Here's how the part is built. I have some questions about the finished solid (model axes, mm). A direction names the side the tool comes from. Round coordinates to 2 decimals unless told otherwise and drop trailing zeros. Write each loop counter-clockwise with the first axis right and the second up, starting at its lowest first coordinate (ties: lowest second). Pieces come first, ordered by that corner, then holes. Notation, with made-up numbers: (21, 15) -> (76, 15) arc R33 ccw to (76, 45) -> close; hole circle Ø3 at (3.25, 70.25). An arc over 180 degrees is marked (long way). Put each result on its own line as item: value. Start each with the question number.
1. Suppose I cut it at A-A (y = 0). Please give me the cut outline in (x, z), then the cut area to 3 significant figures.
2. I need wall thicknesses on probe 1 along X at (y, z) = (0, 2.5); probe 2 along X at (y, z) = (-3.5, -7.5); probe 3 along Z at (x, y) = (7.5, -0.25). Which ranges of each line are inside material? Lowest first, please. Write a range as from..to.
3. Suppose I cut it at D-D (x = 11.5). Please give me the cut outline in (y, z).
4. Suppose I cut it at B-B (z = 0). Please give me the cut outline in (x, y), then the cut area to 3 significant figures.
5. Suppose I cut it at C-C (x = 29). Please give me the cut outline in (y, z), then the cut area to 3 significant figures.
6. For pin 1 (5 mm diameter, centred on x = 8.5, y = -5, fed in from +Z); pin 2 (3 mm diameter, centred on x = 17, z = -2.5, fed in from +Y); pin 3 (5 mm diameter, centred on y = 10, z = -9.5, fed in from +X); pin 4 (2.5 mm diameter, centred on x = 29, y = 0, fed in from +Z), each with a flat end and sliding along its axis, tell me the tip position at first contact or that it passes through.
7. Which directions (+Z, -Z, +X, -X, +Y, -Y) give clear straight access to the entire face, cutting with the end or side of a thin tool? Please do faces 1 (the face through (-4.5, 0, 0)), 2 (the face through (16.22, 3.69, -7.1)).
Autodesk Inventor part; units mm, degrees
ref_plane "Work Plane1" through (17.5, 0, 8) normal (0, 0, 1) x (1, 0, 0)
ref_plane "YZ Plane" through (0, 0, 0) normal (1, 0, 0) x (0, 1, 0)
ref_plane "XZ Plane" through (0, 0, 0) normal (0, 1, 0) x (-1, 0, 0)
sketch "Sketch1" plane through (0, 0, 0) normal (0, 0, 1) x (1, 0, 0)
  line L0 (-4.5, 0) -> (-4.5, 12.5)
  line L1 (-4.5, 12.5) -> (0, 12.5)
  line L2 (0, 12.5) -> (0, 8)
  line L3 (0, 8) -> (35, 8)
  line L4 (35, 8) -> (35, 0)
  line L5 (-4.5, 0) -> (35, 0)
  line L6 (-4, 0) -> (17, 0)
  line L7 (0, -0.98) -> (0, 3.08)
  circle A0 centre (29, 0) radius 2
  dimension "d0" = 16
  dimension "d1" = 25
  dimension "d2" = 4.5
  dimension "d3" = 35
  dimension "d5" = 6
  dimension "d6" = 4
revolve "Body" add sketch "Sketch1" angle 360 about axis through (-4.5, 0, 0) along (1, 0, 0) picked at (28.3903, 0.4694) contours L0 L1 L2 L3 L4 L5 A0 | A0 L5
extrude "Hole" cut sketch "Sketch1" along normal through all both and the other way through all contours A0 L5 | L5 A0
chamfer "Chamfer1" distance 1.6 angle 45 1 edges at (-4.5, -12.5, 0) measured on face at (-3, 12.4595, -1.0058)
chamfer "Chamfer2" distance 3 angle 30 1 edges at (35, -8, 0) measured on face at (11.6667, 7.9741, -0.6437)
ref_plane "Work Plane1" through (17.5, 0, 8) normal (0, 0, 1) x (1, 0, 0)
equation "\"d0\" = NND"
equation "\"d1\" = KOD"
equation "\"d2\" = KOH"
equation "\"d3\" = NLG"
equation "\"d5\" = DIST"
equation "\"d6\" = BOR"
equation "\"d7\" = NND"
equation "\"d9\" = PHH2"
equation "\"d10\" = FAWI2"
equation "\"d16\" = PHH2"
equation "\"d11\" = PHH1"
equation "\"d12\" = FAWI1"
equation "\"d17\" = PHH1"
equation "\"PHH1\" = 3"
equation "\"PHH2\" = 1.6"
equation "\"KOD\" = 25"
equation "\"KOH\" = 4.5"
equation "\"NND\" = 16"
equation "\"FAWI1\" = 30deg"
equation "\"FAWI2\" = 45deg"
equation "\"DIST\" = 6"
equation "\"BOR\" = 4"
equation "\"NLG\" = 35"
properties part number "ISO 2341 - B - 16 x 35" material "Steel"
Verdict:
1. outline: (-4.5, -10.9) -> (-2.9, -12.5) -> (0, -12.5) -> (0, -8) -> (27, -8) -> (27, 8) -> (0, 8) -> (0, 12.5) -> (-2.9, 12.5) -> (-4.5, 10.9) -> close; (31, -8) -> (32, -8) -> (35, -6.27) -> (35, 6.27) -> (32, 8) -> (31, 8) -> close
1. area: 601 mm^2
2. probe 1: x = -4.5..27, 31..35
2. probe 2: x = -4.5..0
2. probe 3: z = -8..8
3. outline: circle Ø16 at (0, 0)
4. outline: (-4.5, -10.9) -> (-2.9, -12.5) -> (0, -12.5) -> (0, -8) -> (32, -8) -> (35, -6.27) -> (35, 6.27) -> (32, 8) -> (0, 8) -> (0, 12.5) -> (-2.9, 12.5) -> (-4.5, 10.9) -> close; hole circle Ø4 at (29, 0)
4. area: 652 mm^2
5. outline: (-2, -7.75) -> (-2, 7.75) arc R8 ccw to start; (2, -7.75) arc R8 ccw to (2, 7.75) -> close
5. area: 138 mm^2
6. pin 1: stops at z = 7.6
6. pin 2: stops at y = 7.94
6. pin 3: stops at x = 0
6. pin 4: passes through
7. face 1: +Z, -Z, -X, +Y, -Y
7. face 2: +X
